CAD build for the part. Positions are in the model's coordinates, mm. A direction names the side the tool comes from. Round coordinates to 2 decimals unless told otherwise and drop trailing zeros. Loops run counter-clockwise (first coordinate to the right, second up) from the corner with the lowest first, then second, coordinate; pieces in that order, holes last.
from build123d import *

# Parameters (mm, degrees)
ESQUISSE1_W             = 134
ESQUISSE1_H             = 134
BOSS_EXTRU_1_DEPTH      = 5
ESQUISSE5_W             = 134
ESQUISSE5_H             = 134
ESQUISSE5_W_2           = 126
ESQUISSE5_H_2           = 126
ENL_V_MAT_EXTRU_1_DEPTH = 3
ESQUISSE6_R             = 1.8
ENL_V_MAT_EXTRU_2_DEPTH = 6
ESQUISSE7_R             = 3
ESQUISSE7_R_2           = 1.8
BOSS_EXTRU_2_DEPTH      = 15
ESQUISSE8_R             = 3
ESQUISSE8_R_2           = 1.8
BOSS_EXTRU_3_DEPTH      = 15
ESQUISSE9_R             = 3
ESQUISSE9_R_2           = 1.8
BOSS_EXTRU_6_DEPTH      = 15
ESQUISSE10_R            = 3
ESQUISSE10_R_2          = 1.8
BOSS_EXTRU_7_DEPTH      = 15


with BuildPart() as part:
    # Esquisse1 → Boss.-Extru.1 (new body)
    with BuildSketch(Plane.XY):
        Rectangle(ESQUISSE1_W, ESQUISSE1_H)
    extrude(amount=BOSS_EXTRU_1_DEPTH)

    # Esquisse5 → Enlèv. mat.-Extru.1 (cut)
    with BuildSketch(Plane.XY):
        Rectangle(ESQUISSE5_W, ESQUISSE5_H)
        Rectangle(ESQUISSE5_W_2, ESQUISSE5_H_2, mode=Mode.SUBTRACT)
    extrude(amount=ENL_V_MAT_EXTRU_1_DEPTH, mode=Mode.SUBTRACT)

    # Esquisse6 → Enlèv. mat.-Extru.2 (cut)
    with BuildSketch(Plane.XY):
        with Locations((57.2, 57.2)):
            Circle(ESQUISSE6_R)
        with Locations((57.2, -57.2)):
            Circle(ESQUISSE6_R)
        with Locations((-57.2, -57.2)):
            Circle(ESQUISSE6_R)
        with Locations((-57.2, 57.2)):
            Circle(ESQUISSE6_R)
    extrude(amount=ENL_V_MAT_EXTRU_2_DEPTH, mode=Mode.SUBTRACT)

    # Esquisse7 → Boss.-Extru.2 (add)
    with BuildSketch(Plane.XY):
        with Locations((57.2, 57.2)):
            Circle(ESQUISSE7_R)
        with Locations((57.2, 57.2)):
            Circle(ESQUISSE7_R_2, mode=Mode.SUBTRACT)
    extrude(amount=BOSS_EXTRU_2_DEPTH)

    # Esquisse8 → Boss.-Extru.3 (add)
    with BuildSketch(Plane.XY):
        with Locations((-57.2, 57.2)):
            Circle(ESQUISSE8_R)
        with Locations((-57.2, 57.2)):
            Circle(ESQUISSE8_R_2, mode=Mode.SUBTRACT)
    extrude(amount=BOSS_EXTRU_3_DEPTH)

    # Esquisse9 → Boss.-Extru.6 (add)
    with BuildSketch(Plane.XY):
        with Locations((-57.2, -57.2)):
            Circle(ESQUISSE9_R)
        with Locations((-57.2, -57.2)):
            Circle(ESQUISSE9_R_2, mode=Mode.SUBTRACT)
    extrude(amount=BOSS_EXTRU_6_DEPTH)

    # Esquisse10 → Boss.-Extru.7 (add)
    with BuildSketch(Plane.XY):
        with Locations((57.2, -57.2)):
            Circle(ESQUISSE10_R)
        with Locations((57.2, -57.2)):
            Circle(ESQUISSE10_R_2, mode=Mode.SUBTRACT)
    extrude(amount=BOSS_EXTRU_7_DEPTH)


solid = part.part
Item 1: Cut at D-D (y = -29.5). List the corners of the cut face in (x, z).
Verdict:
outline: (-67, 3) - (-63, 3) - (-63, 0) - (63, 0) - (63, 3) - (67, 3) - (67, 5) - (-67, 5) - close
Item 2: 3-axis set-ups, long thin cutter, end or side, ignore diameter. For faces 1 (the flat face through (63, -1, 1)), 2 (the cylindrical face through (-54.43, -58.35, 9.93)), 3 (the flat face through (-1, -63, 1)): which of +Z, -Z, +X, -X, +Y, -Y reach the whole face in a straight line?
Verdict:
face 1: -Z, +X, +Y, -Y
face 2: +Z
face 3: -Z, +X, -X, -Y
Item 3: Cut at B-B (x = 57.2). List the corners of the cut face in (y, z), plus the area to 3 significant figures.
Verdict:
outline: (-67, 3) - (-63, 3) - (-63, 0) - (-59, 0) - (-59, 15) - (-60.2, 15) - (-60.2, 5) - (-67, 5) - close; (-55.4, 0) - (55.4, 0) - (55.4, 15) - (54.2, 15) - (54.2, 5) - (-54.2, 5) - (-54.2, 15) - (-55.4, 15) - close; (59, 0) - (63, 0) - (63, 3) - (67, 3) - (67, 5) - (60.2, 5) - (60.2, 15) - (59, 15) - close
area: 658 mm2
Item 4: Flat gauge pins, fed straight in: P1, Ø0.9, axis at y = -2, z = 1, coming from the -X side; P2, Ø0.9, axis at x = -0.5, z = 1, coming from the +Y side; P3, Ø1.5, axis at x = 11, z = 1.5, coming from the -Y side. Where does each tip first touch, or does it go through?
Verdict:
P1: stops at x = -63
P2: stops at y = 63
P3: stops at y = -63
Item 5: Cut at A-A (z = 11.5). List the corners of the cut face in (x, y), plus the area to 3 significant figures.
Verdict:
outline: circle Ø6 at (-57.2, -57.2); circle Ø6 at (-57.2, 57.2); circle Ø6 at (57.2, -57.2); circle Ø6 at (57.2, 57.2); hole circle Ø3.6 at (-57.2, -57.2); hole circle Ø3.6 at (-57.2, 57.2); hole circle Ø3.6 at (57.2, -57.2); hole circle Ø3.6 at (57.2, 57.2)
area: 72.4 mm2
Item 6: Mould opens along X. For faces 4 (the flat face through (-63, -1, 1)), 5 (the cylindrical face through (55.4, -57.12, 7.4)), 6 (the flat face through (-1, 63, 1)), 7 (the cylindrical face through (-56.369, 55.603, 7.395)) say: released by +X, released by -X, zero draft, split by the parting line, or undercut.
Verdict:
face 4: released by -X
face 5: undercut
face 6: zero draft
face 7: undercut
Item 7: Wall check: L1, parallel to Y at x = -57.2, z = 6; L2, parallel to X at y = -56, z = 11.75; L3, parallel to Z at x = -40, y = 22.5. Give the ranges that are in metal, low to high.
Verdict:
L1: y = -60.2 to -59, -55.4 to -54.2, 54.2 to 55.4, 59 to 60.2
L2: x = -59.95 to -58.54, -55.86 to -54.45, 54.45 to 55.86, 58.54 to 59.95
L3: z = 0 to 5
